Input: part model. Units: mm. Frame: model coordinates. A direction names the side the tool comes from. Round coordinates to 2 decimals unless told otherwise and drop trailing zeros. Loops run counter-clockwise (first coordinate to the right, second up) from the corner with the lowest first, then second, coordinate; pieces in that order, holes last. Notation, with made-up numbers: M 75,29 L 88,29 A29 cw 88,65 Z; hole C 35.5,-40 d8. An arc over 180 degrees is marked long. Use one line per item in the form item = value. Start each with the question number.
Q1. Section query A-A, the plane y = 16.5. Output: boundary loops of the cut face in (x, z).
Q2. Section query C-C, the plane x = -16.5. Output: boundary loops of the cut face in (y, z) (3 decimals), and give its area (3 significant figures).
Q3. Section query D-D, the plane y = -13. Output: boundary loops of the cut face in (x, z), and give its area (3 significant figures).
Q4. Section query B-B, the plane z = 3.5. Output: boundary loops of the cut face in (x, y) (3 decimals), and give its area (3 significant figures).
Q5. Access query for faces 5 (the flat face through (48.26, 5, 22)), 6 (the cylindrical face through (44.44, 7.733, 26.692)), 7 (the flat face through (34.226, -28.431, 18.029)), 8 (the flat face through (45, -22.225, 18)), 9 (the flat face through (45, 22.225, 18)). Directions: +Z, -Z, +X, -X, +Y, -Y. A direction counts if a zero-diameter tool reaches every point of the face in a straight line with its end or side. Return the directions, or none.
Q6. Mould query, pull axis Z, two halves, no side actions, for faces 1 (the flat face through (-34.158, -28.374, 18.029)), 2 (the cylindrical face through (44.179, 10.144, 22.571)), 3 (the cylindrical face through (44.721, 3.816, 23.097)), 4 (the flat face through (18.3, 37.3, 35.56)). Classes: pulls with the +Z half, pulls with the -Z half, needs draft (parallel to the pull), parting line crosses it, or undercut.
Q7. Ray query, line 1 along Z through (x, y) = (45, 0); line 2 along Z through (x, y) = (42.5, -7.5); line 3 along Z through (x, y) = (45.25, 8). Return the intervals inside material, ascending.
Q8. First-contact query: P1, Ø10, axis at x = -4.5, z = 17.5, coming from the -Y side; P2, Ø5, axis at y = 6, z = 31.5, coming from the -X side; P3, Ø3.5, axis at y = 0, z = 13.9, coming from the -X side (3 decimals). Flat tips, straight axial feed; report the tip coordinate or a pass-through.
```python
from build123d import *

# Parameters (mm, degrees)
F0_R      = 47.625
F1_DEPTH  = 35.56
F2_R      = 41.275
F3_DEPTH  = 35.561
F5_W      = 44.45
F5_H      = 35.56
F7_R      = 2.2479
F7_R_2    = 4.0005
F8_DEPTH  = 8.2784267637
F10_DEPTH = 35.5610001
F12_DEPTH = 6.35


with BuildPart() as f1:
    # F0 (on Top) → F1 (new body)
    with BuildSketch(Plane.XY):
        Circle(F0_R)
    extrude(amount=F1_DEPTH)

    # F2 (on face) → F3 (cut, through all)
    with BuildSketch(Plane.XY.offset(35.56)):
        Circle(F2_R)
    extrude(amount=-F3_DEPTH, mode=Mode.SUBTRACT)

    # F5 (on offset) → F6 (join, up to the next surface of F1)
    with BuildSketch(Plane.YZ.offset(48.26)):
        with Locations((0, 17.78)):
            Rectangle(F5_W, F5_H)
    extrude(until=Until.NEXT, dir=(-1, 0, 0))

    # F7 (on face) → F8 (cut, through all)
    with BuildSketch(Plane.YZ.offset(48.26)):
        with Locations((0, 29.8958)):
            Circle(F7_R)
        with Locations((-5.6568542495, 27.5526542495)):
            Circle(F7_R)
        with Locations((-8, 21.8958)):
            Circle(F7_R)
        with Locations((-5.6568542495, 16.2389457505)):
            Circle(F7_R)
        with Locations((0, 13.8958)):
            Circle(F7_R)
        with Locations((5.6568542495, 16.2389457505)):
            Circle(F7_R)
        with Locations((8, 21.8958)):
            Circle(F7_R)
        with Locations((5.6568542495, 27.5526542495)):
            Circle(F7_R)
        with Locations((0, 21.8958)):
            Circle(F7_R_2)
    extrude(amount=-F8_DEPTH, mode=Mode.SUBTRACT)

    # F9 (on face) → F10 (cut, through all)
    with BuildSketch(Plane.XY.offset(35.56)):
        Polygon((31.75, -26.3735307648), (-31.75, -26.3735307648), (-65.0275838732, -54.0159679949), (65.0275838732, -54.0159679949), align=None)
    extrude(amount=-F10_DEPTH, mode=Mode.SUBTRACT)

    # F11 (on Top) → F12 (join)
    with BuildSketch(Plane.XY):
        with BuildLine():
            Line((-36.6346153846, -30.4309970363), (-31.75, -26.3735307648))
            ThreePointArc((-31.75, -26.3735307648), (-37.3643754619, 17.536506817), (0, 41.275))
            Line((0, 41.275), (0, 47.625))
            Line((0, 47.625), (-87.4346153846, 47.625))
            Line((-87.4346153846, 47.625), (-87.4346153846, -30.4309970363))
            Line((-87.4346153846, -30.4309970363), (-36.6346153846, -30.4309970363))
        make_face()
    extrude(amount=F12_DEPTH)


solid = f1.part
```
Results found:
q1.outline = M -87.43,0 L -37.83,0 L -37.83,35.56 L -44.68,35.56 L -44.68,6.35 L -87.43,6.35 Z; M 37.83,0 L 48.26,0 L 48.26,35.56 L 37.83,35.56 Z
q2.outline = M 37.834,0 L 47.625,0 L 47.625,6.35 L 44.675,6.35 L 44.675,35.56 L 37.834,35.56 Z
q2.area = 262 mm²
q3.outline = M -87.43,0 L -39.17,0 L -39.17,35.56 L -45.82,35.56 L -45.82,6.35 L -87.43,6.35 Z; M 39.17,0 L 48.26,0 L 48.26,35.56 L 39.17,35.56 Z
q3.area = 824 mm²
q4.outline = M -87.435,-30.431 L -36.635,-30.431 L -31.75,-26.374 A41.275 cw long 31.75,-26.374 L 36.635,-30.431 A47.625 ccw 42.121,-22.225 L 48.26,-22.225 L 48.26,22.225 L 42.121,22.225 A47.625 ccw 0,47.625 L -87.435,47.625 Z
q4.area = 5,090 mm²
q5.face_5 = +Z, -Z, +X, +Y, -Y
q5.face_6 = +X
q5.face_7 = +Z, -Z, -Y
q5.face_8 = +Z, -Z, +X, -Y
q5.face_9 = +Z, -Z, +X, +Y
q6.face_1 = needs draft
q6.face_2 = undercut
q6.face_3 = undercut
q6.face_4 = pulls with the +Z half
q7.line_1 = 0 to 11.65, 16.14 to 17.9, 25.9 to 27.65, 32.14 to 35.56
q7.line_2 = 0 to 14.95, 17.53 to 19.7, 24.09 to 26.27, 28.84 to 35.56
q7.line_3 = 0 to 19.65, 24.14 to 35.56
q8.P1 = 40.17
q8.P2 = -47.5
q8.P3 = -47.625
